```python
from build123d import *

# Parameters (mm, degrees)
SKETCH1_W           = 78.486
SKETCH1_H           = 86.614
SKETCH1_R           = 1.5875
BOSS_EXTRUDE1_DEPTH = 2.54
SKETCH2_R           = 1.27
SKETCH2_W           = 41.275
SKETCH2_H           = 5.08
BOSS_EXTRUDE2_DEPTH = 13.208


with BuildPart() as part:
    # Sketch1 → Boss-Extrude1 (new body)
    with BuildSketch(Plane.XY):
        with Locations((39.243, 43.307)):
            Rectangle(SKETCH1_W, SKETCH1_H)
        with Locations((6.223, 80.1116)):
            Circle(SKETCH1_R, mode=Mode.SUBTRACT)
        with Locations((72.263, 80.1116)):
            Circle(SKETCH1_R, mode=Mode.SUBTRACT)
        with Locations((72.263, 3.9116)):
            Circle(SKETCH1_R, mode=Mode.SUBTRACT)
        with Locations((6.223, 3.9116)):
            Circle(SKETCH1_R, mode=Mode.SUBTRACT)
    extrude(amount=BOSS_EXTRUDE1_DEPTH)

    # Sketch2 → Boss-Extrude2 (add)
    with BuildSketch(Plane.XY.offset(2.54)):
        with Locations((21.082, 10.7569)):
            Circle(SKETCH2_R)
        with Locations((57.404, 7.8105)):
            Circle(SKETCH2_R)
        with Locations((39.243, 67.564)):
            Rectangle(SKETCH2_W, SKETCH2_H)
    extrude(amount=BOSS_EXTRUDE2_DEPTH)


solid = part.part
```
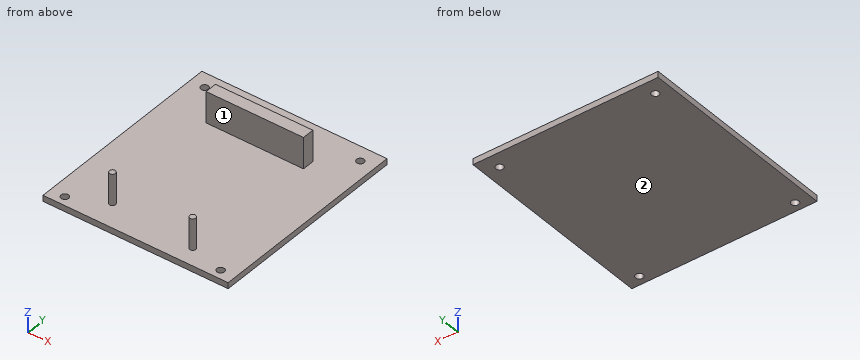
Work out the finished part from the listing and answer in its coordinate system (mm). Face numbers are marked on the shaded views. Coordinates: 2 decimals unless noted, no trailing zeros. Loops run counter-clockwise (first coordinate to the right, second up) from the corner with the lowest first, then second, coordinate; pieces in that order, holes last.
1) Section D-D (z = 6.25) is taken. Give the vertices of the cut face in (x, y).
Results:
outline: (18.61, 65.02) - (59.88, 65.02) - (59.88, 70.1) - (18.61, 70.1) - close; circle Ø2.54 at (21.08, 10.76); circle Ø2.54 at (57.4, 7.81)
2) Section A-A (x = 72) is taken. Give the vertices of the cut face in (y, z).
Results:
outline: (0, 0) - (2.35, 0) - (2.35, 2.54) - (0, 2.54) - close; (5.48, 0) - (78.55, 0) - (78.55, 2.54) - (5.48, 2.54) - close; (81.68, 0) - (86.61, 0) - (86.61, 2.54) - (81.68, 2.54) - close
3) Section C-C (x = 44) is taken. Give the vertices of the cut face in (y, z), plus the area to 3 significant figures.
Results:
outline: (0, 0) - (86.61, 0) - (86.61, 2.54) - (70.1, 2.54) - (70.1, 15.75) - (65.02, 15.75) - (65.02, 2.54) - (0, 2.54) - close
area: 287 mm2
4) Section B-B (y = 69) is taken. Give the vertices of the cut face in (x, z), plus the area to 3 significant figures.
Results:
outline: (0, 0) - (78.49, 0) - (78.49, 2.54) - (59.88, 2.54) - (59.88, 15.75) - (18.61, 15.75) - (18.61, 2.54) - (0, 2.54) - close
area: 745 mm2
5) Consider probe 1 along X at (y, z) = (69.5, 8.75); probe 2 along Z at (x, y) = (9, 48); probe 3 along Y at (x, z) = (52.5, 3.5). Determine where each line is inside the solid, lowest interval first.
Results:
probe 1: x = 18.61 to 59.88
probe 2: z = 0 to 2.54
probe 3: y = 65.02 to 70.1
6) For a pull along Y with two mould halves and no side action, classify the marked faces 1 and 2 as +Y half, -Y half, draft (parallel to the pull), parting line (faces both ways), or undercut.
Results:
face 1: undercut
face 2: draft
7) Flat-ended cylindrical pins translate along their axes: pin 1 (2.5 mm diameter, centred on x = 72.26, y = 80.11, fed in from -Z); pin 2 (2.5 mm diameter, centred on y = 67.5, z = 12.5, fed in from -X); pin 3 (5.5 mm diameter, centred on y = 67.5, z = 9, fed in from +X); pin 4 (6 mm diameter, centred on x = 19.5, z = 6.5, fed in from +Y). Find the tip coordinate at first contact, or state that the pin passes through.
Results:
pin 1: passes through
pin 2: stops at x = 18.61
pin 3: stops at x = 59.88
pin 4: stops at y = 70.1
